from build123d import *

# Parameters (mm, degrees)
MODEL_R             = 2
MODEL_W             = 6
MODEL_H             = 5.5
BOSS_EXTRUDE1_DEPTH = 6


with BuildPart() as part:
    # Model → Boss-Extrude1 (new body)
    with BuildSketch(Plane.XY):
        Polygon((-665.309655483, 302.874496351), (-665.309655483, 339.624496351), (-671.309655483, 339.624496351), (-671.309655483, 345.124496351), (-665.309655483, 345.124496351), (-665.309655483, 452.874496351), (-678.309655483, 452.874496351), (-678.309655483, 458.373843725), (-691.308294267, 458.372538473), (-691.309655483, 452.874496351), (-704.308294267, 452.874496351), (-704.308294267, 458.372538473), (-717.306933052, 458.37123322), (-717.308294267, 452.874496351), (-730.306933052, 452.874496351), (-730.306933052, 458.37123322), (-743.305571836, 458.369927968), (-743.305020076, 452.875099304), (-749.309655483, 452.874496351), (-749.309655483, 416.124496351), (-743.309655483, 416.124496351), (-743.309655483, 410.624496351), (-749.309655483, 410.624496351), (-749.309655483, 302.874496351), (-743.305020081, 302.874496351), (-743.305571836, 297.379717361), (-730.306933052, 297.378412108), (-730.306933052, 302.878412108), (-717.308294267, 302.877106856), (-717.306933052, 297.378412108), (-704.308294267, 297.377106856), (-704.308294267, 302.877106856), (-691.309655483, 302.875801604), (-691.308294267, 297.377106856), (-678.309655483, 297.375801604), (-678.309655483, 302.875801604), align=None)
        with Locations((-710.804492218, 322.87645388)):
            Circle(MODEL_R, mode=Mode.SUBTRACT)
        with Locations((-710.804492218, 432.873034264)):
            Circle(MODEL_R, mode=Mode.SUBTRACT)
        with Locations((-698.309655483, 413.374496351)):
            Rectangle(MODEL_W, MODEL_H, mode=Mode.SUBTRACT)
        with Locations((-686.309655483, 413.374496351)):
            Rectangle(MODEL_W, MODEL_H, mode=Mode.SUBTRACT)
        with Locations((-674.309655483, 413.374496351)):
            Rectangle(MODEL_W, MODEL_H, mode=Mode.SUBTRACT)
        with Locations((-710.309655483, 413.374496351)):
            Rectangle(MODEL_W, MODEL_H, mode=Mode.SUBTRACT)
        with Locations((-722.309655483, 413.374496351)):
            Rectangle(MODEL_W, MODEL_H, mode=Mode.SUBTRACT)
        with Locations((-734.309655483, 413.374496351)):
            Rectangle(MODEL_W, MODEL_H, mode=Mode.SUBTRACT)
        with Locations((-704.309655483, 342.374496351)):
            Rectangle(MODEL_W, MODEL_H, mode=Mode.SUBTRACT)
        with Locations((-692.309655483, 342.374496351)):
            Rectangle(MODEL_W, MODEL_H, mode=Mode.SUBTRACT)
        with Locations((-680.309655483, 342.374496351)):
            Rectangle(MODEL_W, MODEL_H, mode=Mode.SUBTRACT)
        with Locations((-716.309655483, 342.374496351)):
            Rectangle(MODEL_W, MODEL_H, mode=Mode.SUBTRACT)
        with Locations((-728.309655483, 342.374496351)):
            Rectangle(MODEL_W, MODEL_H, mode=Mode.SUBTRACT)
        with Locations((-740.309655483, 342.374496351)):
            Rectangle(MODEL_W, MODEL_H, mode=Mode.SUBTRACT)
    extrude(amount=BOSS_EXTRUDE1_DEPTH)


solid = part.part
Design review of the part built by this model. Coordinates are the model's own, in mm. A direction names the side the tool comes from. Give positions to 0.01 mm unless a question says otherwise; leave off trailing zeros. Loops run counter-clockwise (first coordinate to the right, second up) from the corner with the lowest first, then second, coordinate; pieces in that order, holes last. Notation, with made-up numbers: M -22,68 L 12,68 A12 ccw 12,74 Z; hole C -14.5,7 d9. An arc over 180 degrees is marked long. Write item = value, one per line.
Q1. For faces 5 (the flat face through (-689.31, 413, 3)), 6 (the flat face through (-678.31, 456, 3)), 7 (the flat face through (-671.31, 342, 3)), 8 (the flat face through (-708, 379, 6)), list the 3-axis set-ups (+Z, -Z, +X, -X, +Y, -Y) from which the entire face can be reached by the end or side of a thin tool; tool diameter is ignored.
Output values:
face_5 = +Z, -Z
face_6 = +Z, -Z, +X, +Y
face_7 = +Z, -Z, +X
face_8 = +Z, +X, -X, +Y, -Y
Q2. Draft analysis for pull direction X (two halves, no side actions). For faces 1 (the flat face through (-749.31, 358, 3)), 2 (the flat face through (-746, 410.624, 3)), 3 (the flat face through (-704.308, 456, 3)), 4 (the flat face through (-701.31, 342, 3)), state which applies: +X half, -X half, draft (parallel to the pull), parting line (faces both ways), or undercut.
Output values:
face_1 = -X half
face_2 = draft
face_3 = undercut
face_4 = undercut
Q3. We need section A-A (x = -715.5). Give the boundary of the cut face in (y, z), plus the area to 3 significant figures.
Output values:
outline = M 297.38,0 L 339.62,0 L 339.62,6 L 297.38,6 Z; M 345.12,0 L 458.37,0 L 458.37,6 L 345.12,6 Z
area = 933 mm^2
Q4. Insertion check: pin 1 (1.6 mm diameter, centred on y = 412, z = 1.5, fed in from -X); pin 2 (4 mm diameter, centred on x = -674, y = 374.5, fed in from -Z); pin 3 (3 mm diameter, centred on x = -741.5, z = 3.5, fed in from -Y); pin 4 (1.6 mm diameter, centred on y = 343.5, z = 3.5, fed in from +X). Each pin has a flat end and moves straight along its axis. Give the tip position at first contact, or say it passes through.
Output values:
pin_1 = -743.31
pin_2 = 0
pin_3 = 297.38
pin_4 = -671.31
Q5. We need section C-C (z = 3.7). Count the separate pieces of the cut face and the enclosed holes in it, plus the area to 3 significant figures.
Output values:
separate_pieces = 1
enclosed_holes = 14
area = 12,500 mm^2
Q6. To check wall thickness, follow line 1 (Y direction, x = -681.5, z = 3.7); line 2 (Y direction, x = -743.5, z = 0.3); line 3 (X direction, y = 322, z = 4.55). State the ranges of each line that lie inside material, in increasing order. Write a range as [from, to].
Output values:
line_1 = [297.38, 339.62], [345.12, 458.37]
line_2 = [302.87, 410.62], [416.12, 452.88]
line_3 = [-749.31, -712.6], [-709.01, -665.31]
